Answer from the drawing. Dimensions are ordinates in mm from the lowest x, y and z of the part. Round coordinates to 2 decimals unless told otherwise and drop trailing zeros. Loops run counter-clockwise (first coordinate to the right, second up) from the corner with the lowest first, then second, coordinate; pieces in that order, holes last. Notation, with made-up numbers: (41, -36.75) - (67, -36.75) arc R21 ccw to (67, -28.75) - close; hole circle Ø7 at (-17, -12). An arc over 180 degrees is marked (long way). Write item = value, one per line. Start each with the question number.
1) Section B-B, the plane x = 14 is taken. Determine the outline of the cut face in (y, z), and give its area (3 significant figures).
2) For a pull along X with two mould halves and no side action, classify the marked faces 1, 2 and 3 as released by +X, released by -X, zero draft, split by the parting line, or undercut.
3) Straight lines are drawn through the part: line 1 along X through (y, z) = (3, 24.5); line 2 along X through (y, z) = (7, 28); line 3 along Y through (x, z) = (14, 10.5). For each, find the intervals that lie inside material, in ascending order.
4) Section A-A, the plane z = 65 is taken. Determine the outline of the cut face in (x, y).
5) Section C-C, the plane x = 54.5 is taken. Determine the outline of the cut face in (y, z), and give its area (3 significant figures).
6) Given pin 1 Ø6 at (x, z) = (19, 27.5) entering from -Y; pin 2 Ø11 at (x, y) = (31, 4) entering from +Z, each flat-ended and moving along its own axis, determine where each tip first touches the part or whether it passes through.
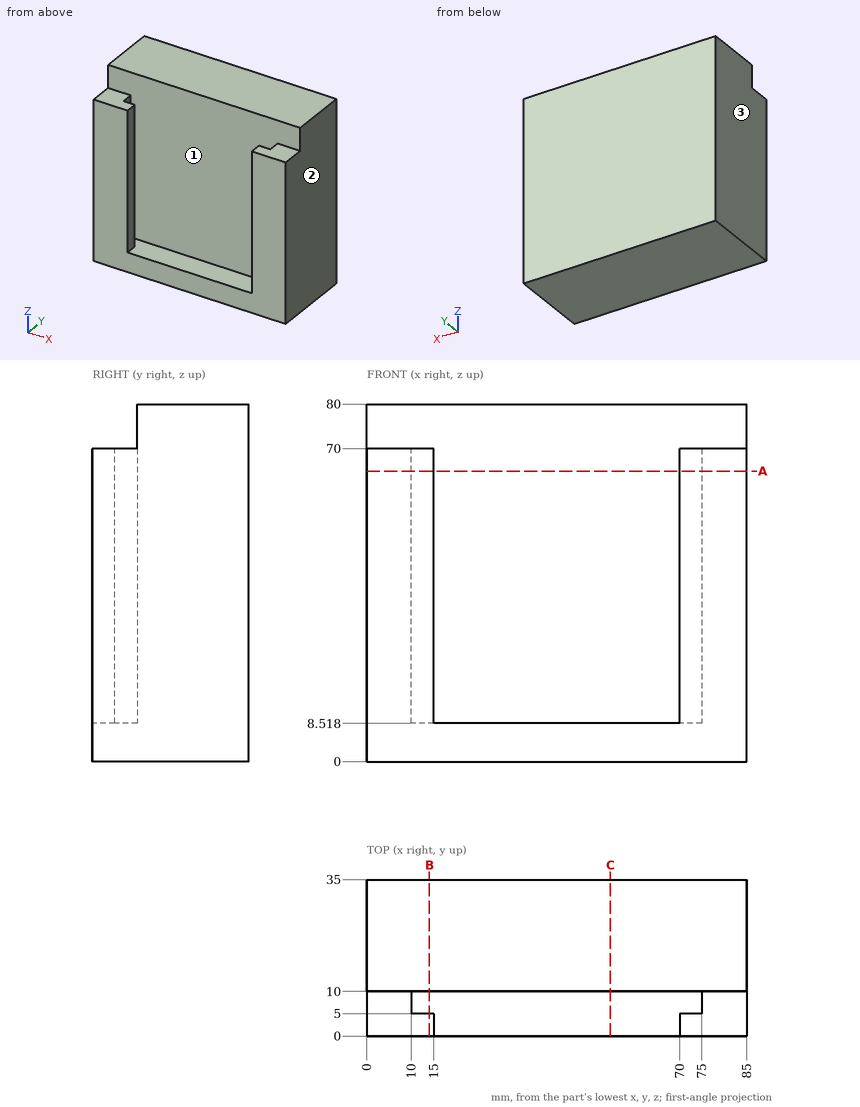
Geometry check:
q1.outline = (0, 0) - (35, 0) - (35, 80) - (10, 80) - (10, 8.52) - (5, 8.52) - (5, 70) - (0, 70) - close
q1.area = 2,390 mm2
q2.face_1 = undercut
q2.face_2 = released by +X
q2.face_3 = released by -X
q3.line_1 = 0 to 15, 70 to 85
q3.line_2 = 0 to 10, 75 to 85
q3.line_3 = 0 to 5, 10 to 35
q4.outline = (0, 0) - (15, 0) - (15, 5) - (10, 5) - (10, 10) - (75, 10) - (75, 5) - (70, 5) - (70, 0) - (85, 0) - (85, 35) - (0, 35) - close
q5.outline = (0, 0) - (35, 0) - (35, 80) - (10, 80) - (10, 8.52) - (0, 8.52) - close
q5.area = 2,090 mm2
q6.pin_1 = 10
q6.pin_2 = 8.52
